Solid Edge part; units mm, degrees
sketch "Sketch1" plane through (0, 0, 0) normal (0, 0, 1) x (1, 0, 0)
  line L0 (-200, -75) -> (200, -75)
  line L1 (200, -75) -> (200, 75)
  line L2 (200, 75) -> (-200, 75)
  line L3 (-200, 75) -> (-200, -75)
extrude "Protrusion1" add sketch "Sketch1" along normal blind 150
sketch "Sketch2" plane through (-200, 0, 75) normal (-1, 0, 0) x (0, -1, 0)
  circle A0 centre (0, 0) radius 60
extrude "Cutout1" cut sketch "Sketch2" against normal up to next
sketch "Sketch3" plane through (0, 0, 150) normal (0, 0, 1) x (0, -1, 0)
  circle A0 centre (0, -170) radius 4.5
  circle A1 centre (0, 170) radius 4.5
extrude "Cutout2" cut sketch "Sketch3" against normal up to next
hole "Hole_1" at (-155, 0, 150) direction (0, 0, -1) diameter 4.917 depth 12 thread major 6 thread length 10
pattern_circular "Pattern1" count 6 over 360 about axis through (-170, 0, 150) along (0, 0, -1) of "Hole_1"
sketch "Sketch4" plane through (0, 0, 150) normal (0, 0, 1) x (0, -1, 0)
  circle A0 centre (0, -170) radius 11
  circle A1 centre (0, -170) radius 8
extrude "CF16_groove" cut sketch "Sketch4" against normal blind 0.7
mirror "Mirror1" about plane through (0, 0, 0) normal (-1, 0, 0) of "Pattern1", "Hole_1", "CF16_groove"
The listing builds one solid part. Answer for the finished solid, in the listing's coordinates (mm). A direction names the side the tool comes from. Round coordinates to 2 decimals unless told otherwise and drop trailing zeros. Write each loop counter-clockwise with the first axis right and the second up, starting at its lowest first coordinate (ties: lowest second). Pieces come first, ordered by that corner, then holes. Notation, with made-up numbers: M 45.25,18 L 63.25,18 A18 ccw 63.25,48 Z; hole C -2,4 d1. An arc over 180 degrees is marked long. Write each question's results on one line, items separated by ' | '. Start each with the question number.
Item 1: Straight lines are drawn through the part: L1, parallel to Y at x = -120.5, z = 54.5; L2, parallel to Y at x = -5, z = 72; L3, parallel to Z at x = 34, y = -28.5. For each, find the intervals that lie inside material, in ascending order. Write a range as [from, to].
Item 2: For faces 1 (the face through (-200, 34, 24)), 2 (the face through (165.61, 0.98, 142.52)), determine the directions among +Z, -Z, +X, -X, +Y, -Y from which every point of the face is accessible in a straight line to the end or side of a thin tool.
Item 3: A flat-ended cylindrical pin translates along its axis: pin 1 Ø1.5 at (x, y) = (154, 1) entering from +Z. Find the tip coordinate at first contact, or state that the pin passes through.
Item 4: A cutting plane is placed at C-C on x = 53.5. Write down the section's boundary in (y, z), and give its area (3 significant figures).
Item 5: A cutting plane is placed at D-D on x = -170. Write down the section's boundary in (y, z).
Item 6: A cutting plane is placed at A-A on y = 36. Write down the section's boundary in (x, z), and give its area (3 significant figures).
Item 7: For a pull along Z with two mould halves and no side action, classify faces 3 (the face through (-2.8, 13.007, 16.427)), 4 (the face through (200, -34, 24)), 5 (the face through (-3, 1, 0)), 6 (the face through (-166.6, -3.4, 150)) as pulls with the +Z half, pulls with the -Z half, needs draft (parallel to the pull), parting line crosses it, or undercut.
Item 8: A cutting plane is placed at B-B on z = 75. Write down the section's boundary in (x, y), and give its area (3 significant figures).
Check sheet entries:
1) L1: [-75, -56.39], [56.39, 75] | L2: [-75, -59.92], [59.92, 75] | L3: [0, 22.2], [127.8, 150]
2) face 1: +Z, -Z, -X, +Y, -Y | face 2: +Z
3) pin 1: z = 138
4) outline: M -75,0 L 75,0 L 75,150 L -75,150 Z; hole C 0,75 d120 | area: 11,200 mm²
5) outline: M -75,0 L 75,0 L 75,150 L 11,150 L 11,149.3 L 8,149.3 L 8,150 L 4.5,150 L 4.5,134.83 A60 cw long -4.5,134.83 L -4.5,150 L -8,150 L -8,149.3 L -11,149.3 L -11,150 L -75,150 Z
6) outline: M -200,0 L 200,0 L 200,27 L -200,27 Z; M -200,123 L 200,123 L 200,150 L -200,150 Z | area: 21,600 mm²
7) face 3: undercut | face 4: needs draft | face 5: pulls with the -Z half | face 6: pulls with the +Z half
8) outline: M -200,-75 L 200,-75 L 200,-60 L -200,-60 Z; M -200,60 L 200,60 L 200,75 L -200,75 Z | area: 12,000 mm²
